Autodesk Inventor part; units mm, degrees
ref_plane "YZ Plane" through (0, 0, 0) normal (1, 0, 0) x (0, 1, 0)
ref_plane "XZ Plane" through (0, 0, 0) normal (0, 1, 0) x (-1, 0, 0)
ref_plane "XY Plane" through (0, 0, 0) normal (0, 0, 1) x (1, 0, 0)
sketch "Sketch1" plane through (0, 0, 0) normal (0, 1, 0) x (-1, 0, 0)
  line L0 (41.25, -2.25) -> (28.75, -2.25) construction
  line L1 (28.75, -2.25) -> (28.75, -14.75) construction
  line L2 (28.75, -14.75) -> (41.25, -14.75) construction
  line L3 (41.25, -14.75) -> (41.25, -2.25) construction
  line L4 (56.9183, -8.5) -> (8.3915, -8.5) construction
  line L5 (0, -17) -> (105, -17) construction
  line L6 (0, 0) -> (0, -51) construction
  line L7 (0, -34) -> (105, -34) construction
  line L8 (105, -51) -> (105, 0) construction
  line L9 (35, 19) -> (35, -51) construction
  line L10 (56.8064, -25.5) -> (17, -25.5) construction
  line L11 (28.75, -19.25) -> (28.75, -31.75) construction
  line L12 (41.25, -19.25) -> (28.75, -19.25) construction
  line L13 (41.25, -31.75) -> (41.25, -19.25) construction
  line L14 (28.75, -31.75) -> (41.25, -31.75) construction
  line L15 (28.75, -36.25) -> (28.75, -48.75) construction
  line L16 (41.25, -36.25) -> (28.75, -36.25) construction
  line L17 (41.25, -48.75) -> (41.25, -36.25) construction
  line L18 (28.75, -48.75) -> (41.25, -48.75) construction
  line L19 (56.3008, -42.5) -> (16.5498, -42.5) construction
  arc A0 (53.45, -12.2) -> (53.45, -21.8) centre (53.45, -17) ccw
  arc A1 (92, -21.8) -> (92, -12.2) centre (92, -17) ccw
  arc A2 (53.45, -29.2) -> (53.45, -38.8) centre (53.45, -34) ccw construction
  arc A3 (92, -38.8) -> (92, -29.2) centre (92, -34) ccw construction
  line L20 (53.45, -12.2) -> (92, -12.2)
  line L21 (53.45, -21.8) -> (92, -21.8)
  line L22 (53.45, -29.2) -> (92, -29.2) construction
  line L23 (53.45, -38.8) -> (92, -38.8) construction
  arc A4 (16.15, -38.6) -> (16.15, -29.4) centre (16.15, -34) ccw construction
  line L24 (103.5, -49.5) -> (103.5, -1.5) construction
  line L25 (1.5, -1.5) -> (1.5, -49.5) construction
  arc A5 (14, -29.4) -> (14, -38.6) centre (14, -34) ccw construction
  arc A6 (14, -12.4) -> (14, -21.6) centre (14, -17) ccw construction
  line L26 (16.15, -38.6) -> (14, -38.6) construction
  line L27 (14, -29.4) -> (16.15, -29.4) construction
  line L28 (14, -21.6) -> (16.15, -21.6) construction
  line L29 (16.15, -12.4) -> (14, -12.4) construction
  arc A7 (16.15, -21.6) -> (16.15, -12.4) centre (16.15, -17) ccw construction
  arc A8 (96.3, -51) -> (93, -47.7) centre (93, -51) ccw construction
  arc A9 (53.45, -47.7) -> (50.15, -51) centre (53.45, -51) ccw construction
  arc A10 (97.5596, -49.5) -> (93, -46.2) centre (93, -51) ccw construction
  line L30 (93, -46.2) -> (53.45, -46.2) construction
  line L31 (96.3, -51) -> (105, -51) construction
  line L32 (93, -47.7) -> (53.45, -47.7) construction
  line L33 (105, -49.5) -> (97.5596, -49.5) construction
  arc A11 (53.45, -46.2) -> (48.8904, -49.5) centre (53.45, -51) ccw construction
  arc A12 (48.8904, -1.5) -> (53.45, -4.8) centre (53.45, 0) ccw construction
  arc A13 (50.15, 0) -> (53.45, -3.3) centre (53.45, 0) ccw construction
  line L34 (93, -3.3) -> (53.45, -3.3) construction
  line L35 (93, -4.8) -> (53.45, -4.8) construction
  line L36 (97.5596, -1.5) -> (105, -1.5) construction
  line L37 (105, 0) -> (96.3, 0) construction
  arc A14 (93, -3.3) -> (96.3, 0) centre (93, 0) ccw construction
  arc A15 (93, -4.8) -> (97.5596, -1.5) centre (93, 0) ccw construction
  arc A16 (20.45, -51) -> (17.15, -47.7) centre (17.15, -51) ccw construction
  arc A17 (12, -47.7) -> (8.7, -51) centre (12, -51) ccw construction
  line L38 (17.15, -46.2) -> (12, -46.2) construction
  line L39 (17.15, -47.7) -> (12, -47.7) construction
  arc A18 (12, -46.2) -> (7.4404, -49.5) centre (12, -51) ccw construction
  arc A19 (21.7096, -49.5) -> (17.15, -46.2) centre (17.15, -51) ccw construction
  line L40 (48.8904, -49.5) -> (21.7096, -49.5) construction
  line L41 (7.4404, -49.5) -> (0, -49.5) construction
  line L42 (0, -51) -> (8.7, -51) construction
  line L43 (20.45, -51) -> (50.15, -51) construction
  line L44 (17.15, -4.8) -> (12, -4.8) construction
  line L45 (17.15, -3.3) -> (12, -3.3) construction
  arc A20 (8.7, 0) -> (12, -3.3) centre (12, 0) ccw construction
  arc A21 (17.15, -3.3) -> (20.45, 0) centre (17.15, 0) ccw construction
  arc A22 (7.4404, -1.5) -> (12, -4.8) centre (12, 0) ccw construction
  arc A23 (17.15, -4.8) -> (21.7096, -1.5) centre (17.15, 0) ccw construction
  line L46 (50.15, 0) -> (20.45, 0) construction
  line L47 (8.7, 0) -> (0, 0) construction
  line L48 (0, -1.5) -> (7.4404, -1.5) construction
  line L49 (21.7096, -1.5) -> (48.8904, -1.5) construction
  line L50 (113, 2) -> (-20, 2) construction
  line L51 (-20, 2) -> (-20, -53) construction
  line L52 (-20, -53) -> (113, -53) construction
  line L53 (113, -53) -> (113, 2) construction
  arc A24 (92, -23.3) -> (92, -10.7) centre (92, -17) ccw
  arc A25 (53.45, -10.7) -> (53.45, -23.3) centre (53.45, -17) ccw
  line L54 (92, -10.7) -> (53.45, -10.7)
  line L55 (53.45, -23.3) -> (92, -23.3)
  point P0 (35, -8.5)
  point P1 (35, -42.5)
  point P2 (35, -25.5)
  dimension "d0" = 12.5
  dimension "d1" = 12.5
  dimension "d2" = 17
  dimension "d3" = 35
  dimension "d4" = 105
  dimension "d5" = 17
  dimension "d6" = 17
  dimension "d7" = 9.6
  dimension "d8" = 1.5
  dimension "d9" = 1.5
  dimension "d10" = 4.6
  dimension "d11" = 1.5
  dimension "d12" = 1.5
  dimension "d13" = 1.5
  dimension "d14" = 17
  dimension "d15" = 17
  dimension "d16" = 12
  dimension "d17" = 13
  dimension "d18" = 12.2
  dimension "d19" = 11.6
  dimension "d20" = 12.6
  dimension "d21" = 12
  dimension "d22" = 12.5
  dimension "d23" = 2
  dimension "d24" = 8
  dimension "d25" = 20
  dimension "d26" = 1.5
extrude "Extrusion1" add sketch "Sketch1" along normal blind 9.5 contours L20 A1 L21 A0
extrude "Extrusion2" add sketch "Sketch1" along normal blind 4
chamfer "Chamfer1" distance 0.5 angle 45 4 edges at (-72.725, 9.5, -12.2) (-48.65, 9.5, -17) (-72.725, 9.5, -21.8) (-96.8, 9.5, -17)
hole "Hole1" at (-35, 0, -8.5) at (0, 0, -17) at (-35, 0, -42.5) at (-35, 0, -25.5) at (-92, 0, -17) at (-53.45, 0, -17) direction (0, 1, 0) diameter 4 end through all counterbore diameter 6 counterbore depth 3
properties part number "Large_retainer"
Design review of the part built by this model. Coordinates are the model's own, in mm. A direction names the side the tool comes from. Give positions to 0.01 mm unless a question says otherwise; leave off trailing zeros. Write each loop counter-clockwise with the first axis right and the second up, starting at its lowest first coordinate (ties: lowest second). Pieces come first, ordered by that corner, then holes. Notation, with made-up numbers: M 42,-38 L 99,-38 A30 cw 99,-14 Z; hole C 44,28.25 d11. An arc over 180 degrees is marked long. Answer as a JSON object with one key per item and string values. Group by question number.
1) We need section D-D (y = 1.5). Give the boundary of the cut face in (x, z), and give its area (3 significant figures).
2) We need section A-A (z = -17). Give the boundary of the cut face in (x, y).
3) Mouldability with a two-part tool opening along X and no side actions: class faces 4 (the face through (-50.52, 1.52, -16.35)), 5 (the face through (-72, 2, -23.3)), 6 (the face through (-96.44, 9.36, -16.9)), 7 (the face through (-49.01, 9.36, -17.1)) as released by +X, released by -X, zero draft, split by the parting line, or undercut.
4) For line 1 along X through (y, z) = (1.25, -17); line 2 along X through (y, z) = (9, -17); line 3 along Z through (x, y) = (-92, 1.3), list the stretches that pass through material, from the lowest coordinate up.
5) Tool access review of faces 1 (the face through (-51, 3, -18)), 2 (the face through (-72, 6, -21.8)), 3 (the face through (-96.8, 6.5, -16.9)): name each direction out of +Z, -Z, +X, -X, +Y, -Y from which nothing blocks a thin tool from reaching the whole face with its end or side.
6) We need section B-B (y = 7). Give the boundary of the cut face in (x, z), and give its area (3 significant figures).
7) We need section C-C (x = -62). Give the boundary of the cut face in (y, z).
8) Clearance check with flat-ended pins moving along their axes: pin 1 Ø4 at (x, y) = (-78.5, 7.5) entering from -Z; pin 2 Ø3 at (x, z) = (-53.45, -17) entering from -Y; pin 3 Ø5 at (x, z) = (-92, -17) entering from -Y; pin 4 Ø1.5 at (x, y) = (-69.5, 6.5) entering from +Z. State where each tip first meets the part, or that it passes through.
Answer key:
{
 "1": {"outline": "M -92,-23.3 L -53.45,-23.3 A6.3 ccw -53.45,-10.7 L -92,-10.7 A6.3 ccw Z; hole C -92,-17 d6; hole C -53.45,-17 d6", "area": "554 mm²"},
 "2": {"outline": "M -98.3,0 L -95,0 L -95,3 L -94,3 L -94,9.5 L -96.3,9.5 L -96.8,9 L -96.8,4 L -98.3,4 Z; M -90,3 L -89,3 L -89,0 L -56.45,0 L -56.45,3 L -55.45,3 L -55.45,9.5 L -90,9.5 Z; M -51.45,3 L -50.45,3 L -50.45,0 L -47.15,0 L -47.15,4 L -48.65,4 L -48.65,9 L -49.15,9.5 L -51.45,9.5 Z"},
 "3": {"face 4": "undercut", "face 5": "zero draft", "face 6": "released by -X", "face 7": "released by +X"},
 "4": {"line 1": "x = -98.3 to -95, -89 to -56.45, -50.45 to -47.15", "line 2": "x = -96.8 to -94, -90 to -55.45, -51.45 to -48.65", "line 3": "z = -23.3 to -20, -14 to -10.7"},
 "5": {"face 1": "-Y", "face 2": "-Z, +X, -X, +Y", "face 3": "-X, +Y"},
 "6": {"outline": "M -92,-21.8 L -53.45,-21.8 A4.8 ccw -53.45,-12.2 L -92,-12.2 A4.8 ccw Z; hole C -92,-17 d4; hole C -53.45,-17 d4", "area": "417 mm²"},
 "7": {"outline": "M 0,-23.3 L 4,-23.3 L 4,-21.8 L 9,-21.8 L 9.5,-21.3 L 9.5,-12.7 L 9,-12.2 L 4,-12.2 L 4,-10.7 L 0,-10.7 Z"},
 "8": {"pin 1": "stops at z = -21.8", "pin 2": "passes through", "pin 3": "stops at y = 3", "pin 4": "stops at z = -12.2"}
}
